from build123d import *

# Parameters (mm, degrees)
SKETCH1_R                = 0.95
BOSS_EXTRUDE1_DEPTH      = 2.55
BOSS_EXTRUDE2_DEPTH      = 0.975
BOSS_EXTRUDE2_DEPTH_BACK = 3.525
SKETCH3_R                = 4.135
CUT_EXTRUDE1_DEPTH       = 1.95
SKETCH4_R                = 4.865
BOSS_EXTRUDE3_DEPTH      = 1.9
SKETCH5_R                = 3.125
CUT_EXTRUDE2_DEPTH       = 3.49


with BuildPart() as part:
    # Sketch1 → Boss-Extrude1 (new body)
    with BuildSketch(Plane(origin=(0, 0, 0), x_dir=(1, 0, 0), z_dir=(0, 1, 0))):
        with BuildLine():
            Line((0, 12.78), (25.28, 10))
            ThreePointArc((25.28, 10), (28.89, 6.39), (25.28, 2.78))
            Line((25.28, 2.78), (0, 0))
            Line((0, 0), (-25.28, 2.78))
            ThreePointArc((-25.28, 2.78), (-28.89, 6.39), (-25.28, 10))
            Line((-25.28, 10), (0, 12.78))
        make_face()
        with Locations(Location((25.28, 6.39, 0), (0, 0, 270))):
            Circle(SKETCH1_R, mode=Mode.SUBTRACT)
        with Locations(Location((22.18, 6.39, 0), (0, 0, 270))):
            Circle(SKETCH1_R, mode=Mode.SUBTRACT)
        with Locations(Location((19.08, 6.39, 0), (0, 0, 270))):
            Circle(SKETCH1_R, mode=Mode.SUBTRACT)
        with Locations(Location((15.98, 6.39, 0), (0, 0, 270))):
            Circle(SKETCH1_R, mode=Mode.SUBTRACT)
        with Locations(Location((12.88, 6.39, 0), (0, 0, 270))):
            Circle(SKETCH1_R, mode=Mode.SUBTRACT)
        with Locations(Location((-12.88, 6.39, 0), (0, 0, 90))):
            Circle(SKETCH1_R, mode=Mode.SUBTRACT)
        with Locations(Location((-15.98, 6.39, 0), (0, 0, 90))):
            Circle(SKETCH1_R, mode=Mode.SUBTRACT)
        with Locations(Location((-19.08, 6.39, 0), (0, 0, 90))):
            Circle(SKETCH1_R, mode=Mode.SUBTRACT)
        with Locations(Location((-22.18, 6.39, 0), (0, 0, 90))):
            Circle(SKETCH1_R, mode=Mode.SUBTRACT)
        with Locations(Location((-25.28, 6.39, 0), (0, 0, 90))):
            Circle(SKETCH1_R, mode=Mode.SUBTRACT)
    extrude(amount=BOSS_EXTRUDE1_DEPTH)

    # Sketch2 → Boss-Extrude2 (add, two sides: drawn at the far end of the back side and taken through both)
    with BuildSketch(Plane(origin=(0, 2.55, 0), x_dir=(1, 0, 0), z_dir=(0, 1, 0)).offset(-BOSS_EXTRUDE2_DEPTH_BACK)):
        Polygon((-9.075, 11.782037184), (-9.075, 0.997962816), (0, 0), (9.075, 0.997962816), (9.075, 11.782037184), (0, 12.78), align=None)
    extrude(amount=BOSS_EXTRUDE2_DEPTH + BOSS_EXTRUDE2_DEPTH_BACK)

    # Sketch3 → Cut-Extrude1 (cut)
    with BuildSketch(Plane.XZ.offset(0.975)):
        with Locations(Location((0, -6.39, 0), (0, 0, 270))):
            Circle(SKETCH3_R)
    extrude(amount=-CUT_EXTRUDE1_DEPTH, mode=Mode.SUBTRACT)

    # Sketch4 → Boss-Extrude3 (add)
    with BuildSketch(Plane(origin=(0, 3.525, 0), x_dir=(1, 0, 0), z_dir=(0, 1, 0))):
        with Locations(Location((0, 6.39, 0), (0, 0, 90))):
            Circle(SKETCH4_R)
    extrude(amount=BOSS_EXTRUDE3_DEPTH)

    # Sketch5 → Cut-Extrude2 (cut)
    with BuildSketch(Plane(origin=(0, 5.425, 0), x_dir=(1, 0, 0), z_dir=(0, 1, 0))):
        with Locations(Location((0, 6.39, 0), (0, 0, 270))):
            Circle(SKETCH5_R)
    extrude(amount=-CUT_EXTRUDE2_DEPTH, mode=Mode.SUBTRACT)


solid = part.part
The model under review builds one solid part; all positions refer to its coordinate system, in mm. A direction names the side the tool comes from. Give positions to 0.01 mm unless a question says otherwise; leave off trailing zeros. Loops run counter-clockwise (first coordinate to the right, second up) from the corner with the lowest first, then second, coordinate; pieces in that order, holes last. Notation, with made-up numbers: (-39, 12) -> (-31, 12) arc R21 ccw to (-31, 34) -> close; hole circle Ø9 at (6.5, 58). An arc over 180 degrees is marked (long way). Put each result on its own line as item: value. Start each with the question number.
1. We need section C-C on x = -15.98. State the section outline as (y, z) points.
2. Clearance check with flat-ended pins moving along their axes: P1, Ø1.5, axis at x = 19.08, z = -6.39, coming from the +Y side; P2, Ø0.5, axis at y = -0.5, z = -5, coming from the +X side (3 decimals); P3, Ø1, axis at x = 18.5, z = -7.5, coming from the +Y side; P4, Ø5.5, axis at x = 0, z = -6.39, coming from the +Y side (3 decimals). State where each tip first meets the part, or that it passes through.
3. We need section B-B on z = -8.25. State the section outline as (x, y) points (3 decimals), then the cut area to 3 significant figures.
4. We need section D-D on x = -5.5. State the section outline as (y, z) points (3 decimals).
5. Mouldability with a two-part tool opening along Z and no side actions: class faces 1 (the face through (0, 0.975, -6)), 2 (the face through (-28.89, 1.26, -6.31)), 3 (the face through (-9.075, 3, -6)) as released by +Z, released by -Z, zero draft, split by the parting line, or undercut.
6. We need section A-A on x = 22.18. State the section outline as (y, z) points.
7. Wall thickness on probe 1 along Y at (x, z) = (14.5, -8.5); probe 2 along Y at (x, z) = (-7, -2.25) (3 decimals); probe 3 along Z at (x, y) = (-12.88, 1.15): over which ranges is each line inside the solid? List them lowest first.
8. For faces 4 (the face through (17, 0, -5)), 5 (the face through (0.14, 3.7, -9.51)), 6 (the face through (9.075, 3, -6)), 7 (the face through (-19, 0, -5)), list the 3-axis set-ups (+Z, -Z, +X, -X, +Y, -Y) from which the entire face can be reached by the end or side of a thin tool; tool diameter is ignored.
Determined:
1. outline: (0, -11.02) -> (2.55, -11.02) -> (2.55, -7.34) -> (0, -7.34) -> close; (0, -5.44) -> (2.55, -5.44) -> (2.55, -1.76) -> (0, -1.76) -> close
2. P1: through
2. P2: x = 9.075
2. P3: y = 2.55
2. P4: y = 1.935
3. outline: (-28.374, 0) -> (-9.075, 0) -> (-9.075, -0.975) -> (-3.693, -0.975) -> (-3.693, 0.975) -> (3.693, 0.975) -> (3.693, -0.975) -> (9.075, -0.975) -> (9.075, 0) -> (28.374, 0) -> (28.374, 2.55) -> (9.075, 2.55) -> (9.075, 3.525) -> (4.495, 3.525) -> (4.495, 5.425) -> (2.511, 5.425) -> (2.511, 1.935) -> (-2.511, 1.935) -> (-2.511, 5.425) -> (-4.495, 5.425) -> (-4.495, 3.525) -> (-9.075, 3.525) -> (-9.075, 2.55) -> (-28.374, 2.55) -> close
3. area: 165 mm^2
4. outline: (-0.975, -12.175) -> (3.525, -12.175) -> (3.525, -0.605) -> (-0.975, -0.605) -> close
5. face 1: undercut
5. face 2: split by the parting line
5. face 3: zero draft
6. outline: (0, -10.34) -> (2.55, -10.34) -> (2.55, -7.34) -> (0, -7.34) -> close; (0, -5.44) -> (2.55, -5.44) -> (2.55, -2.44) -> (0, -2.44) -> close
7. probe 1: 0 to 2.55
7. probe 2: -0.975 to 3.525
7. probe 3: -11.36 to -7.34, -5.44 to -1.42
8. face 4: +Z, -Z, +X, -Y
8. face 5: +Y
8. face 6: +Z, -Z, +X, +Y
8. face 7: +Z, -Z, -X, -Y
